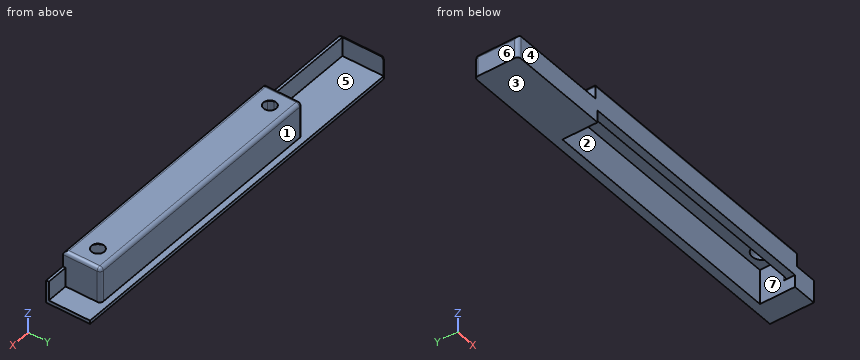
```python
from build123d import *

# Parameters (mm, degrees)
CROQUIS1_W                                   = 220
CROQUIS1_H                                   = 25
SALIENTE_EXTRUIR1_DEPTH                      = 2
SALIENTE_EXTRUIR2_DEPTH                      = 11
SALIENTE_EXTRUIR3_DEPTH                      = 7
CROQUIS5_W                                   = 150
CROQUIS5_H                                   = 20
SALIENTE_EXTRUIR4_DEPTH                      = 2
REDONDEO2_R                                  = 2
REDONDEO3_R                                  = 2
REDONDEO4_R                                  = 2
CROQUIS7_W                                   = 147
CROQUIS7_H                                   = 20
CORTAR_EXTRUIR1_DEPTH                        = 2
CROQUIS10_W                                  = 150
CROQUIS10_H                                  = 1.5
SALIENTE_EXTRUIR8_DEPTH                      = 15
CROQUIS11_R                                  = 2.25
CORTAR_EXTRUIR2_DEPTH                        = 15
REFRENTADO_PARA_TORNILLO_TAP_N_CON_C_2_COUNT = 2
REFRENTADO_PARA_TORNILLO_TAP_N_CON_C_2_PITCH = 128
REDONDEO5_R                                  = 2
CROQUIS14_W                                  = 147
CROQUIS14_H                                  = 3
SALIENTE_EXTRUIR9_DEPTH                      = 13
REDONDEO6_R                                  = 2


with BuildPart() as part:
    # Croquis1 → Saliente-Extruir1 (new body)
    with BuildSketch(Plane.XY):
        with Locations((-129.544939143, 51.184210526)):
            Rectangle(CROQUIS1_W, CROQUIS1_H)
    extrude(amount=SALIENTE_EXTRUIR1_DEPTH)

    # Croquis3 → Saliente-Extruir2 (add)
    with BuildSketch(Plane.XY.offset(2)):
        Polygon((-239.544939143, 63.684210526), (-239.544939143, 38.684210526), (-180.544939143, 38.684210526), (-180.544939143, 58.684210526), (-33.544939143, 58.684210526), (-33.544939143, 38.684210526), (-19.544939143, 38.684210526), (-19.544939143, 40.184210526), (-32.044939143, 40.184210526), (-32.044939143, 60.184210526), (-182.044939143, 60.184210526), (-182.044939143, 40.184210526), (-238.044939143, 40.184210526), (-238.044939143, 63.684210526), align=None)
    extrude(amount=SALIENTE_EXTRUIR2_DEPTH)

    # Croquis4 → Saliente-Extruir3 (add)
    with BuildSketch(Plane.XY.offset(13)):
        Polygon((-182.044939143, 40.184210526), (-180.544939143, 40.184210526), (-180.544939143, 40.470961068), (-180.544939143, 58.684210526), (-33.544939143, 58.684210526), (-33.544939143, 40.470961068), (-33.544939143, 40.184210526), (-32.044939143, 40.184210526), (-32.044939143, 40.470961068), (-32.044939143, 60.184210526), (-182.044939143, 60.184210526), align=None)
    extrude(amount=SALIENTE_EXTRUIR3_DEPTH)

    # Croquis5 → Saliente-Extruir4 (add)
    with BuildSketch(Plane.XY.offset(20)):
        with Locations((-107.044939143, 50.184210526)):
            Rectangle(CROQUIS5_W, CROQUIS5_H)
    extrude(amount=SALIENTE_EXTRUIR4_DEPTH)

    # Redondeo2
    redondeo2_edges = [part.edges().sort_by_distance(p)[0] for p in [
        (-239.544939143, 63.684210526, 6.5),
    ]]
    fillet(redondeo2_edges, radius=REDONDEO2_R)

    # Redondeo3
    # the kernel refuses this fillet: 2 mm, written as the material it takes off along each edge
    with BuildSketch(Plane(origin=(-239.544939143, 61.684210526, 13), x_dir=(1, 0, 0), z_dir=(0, -1, 0))) as redondeo3_piece_1:
        with BuildLine():
            CenterArc((REDONDEO3_R, -REDONDEO3_R), REDONDEO3_R, 90, 90)
            Line((0, -REDONDEO3_R), (0, 0))
            Line((0, 0), (REDONDEO3_R, 0))
        make_face()
    extrude(amount=28, mode=Mode.SUBTRACT)
    with BuildSketch(Plane(origin=(-237.544939143, 61.684210526, 13), x_dir=(0.7793111641702657, -0.6266371433290445, 0), z_dir=(-0.6266371433290445, -0.7793111641702657, 0))) as redondeo3_piece_2:
        with BuildLine():
            CenterArc((2 - REDONDEO3_R, -REDONDEO3_R), REDONDEO3_R, 0, 90)
            Line((2 - REDONDEO3_R, 0), (2, 0))
            Line((2, 0), (2, -REDONDEO3_R))
        make_face()
    revolve(axis=Axis((-237.544939143, 61.684210526, 13), (0, 0, 1)), revolution_arc=218.802450559, mode=Mode.SUBTRACT)

    # Redondeo4
    # the kernel refuses this fillet: 2 mm, written as the material it takes off along each edge
    with BuildSketch(Plane(origin=(-239.544939143, 38.684210526, -5), x_dir=(0, 1, 0), z_dir=(0, 0, 1))) as redondeo4_piece_1:
        with BuildLine():
            CenterArc((REDONDEO4_R, -REDONDEO4_R), REDONDEO4_R, 90, 90)
            Line((0, -REDONDEO4_R), (0, 0))
            Line((0, 0), (REDONDEO4_R, 0))
        make_face()
    extrude(amount=21, mode=Mode.SUBTRACT)

    # Croquis7 → Cortar-Extruir1 (cut)
    with BuildSketch(Plane.XY.offset(2)):
        with Locations((-107.044939143, 48.684210526)):
            Rectangle(CROQUIS7_W, CROQUIS7_H)
    extrude(amount=-CORTAR_EXTRUIR1_DEPTH, mode=Mode.SUBTRACT)

    # Croquis10 → Saliente-Extruir8 (add)
    with BuildSketch(Plane.XY.offset(22)):
        with Locations((-107.044939143, 39.434210526)):
            Rectangle(CROQUIS10_W, CROQUIS10_H)
    extrude(amount=-SALIENTE_EXTRUIR8_DEPTH)

    # Croquis11 → Cortar-Extruir2 (cut)
    with BuildSketch(Plane.XY.offset(22)):
        with Locations((-171.044939143, 50.184210526)):
            Circle(CROQUIS11_R)
        with Locations((-43.044939143, 50.184210526)):
            Circle(CROQUIS11_R)
    extrude(amount=-CORTAR_EXTRUIR2_DEPTH, mode=Mode.SUBTRACT)

    # Croquis12 → Refrentado para tornillo tapón con cabeza plana de clavija de M51 (revolve, cut)
    with BuildSketch(Plane(origin=(-171.044939143, 50.184210526, 20), x_dir=(0, 1, 0), z_dir=(1, 0, 0))):
        Polygon((0, 0), (0, 2), (2.9, 2), (2.9, 2.7), (5.6, 0), align=None)
    refrentado_para_tornillo_tap_n_con_cabez = revolve(axis=Axis((-171.044939143, 50.184210526, 13.65), (0, 0, 1)), mode=Mode.SUBTRACT)

    # Refrentado para tornillo tap_n con c 2: Refrentado para tornillo tapón con cabeza plana de clavija de M51 ×2
    with Locations(*[(i * REFRENTADO_PARA_TORNILLO_TAP_N_CON_C_2_PITCH, 0, 0) for i in range(1, REFRENTADO_PARA_TORNILLO_TAP_N_CON_C_2_COUNT)]):
        add(refrentado_para_tornillo_tap_n_con_cabez, mode=Mode.SUBTRACT)

    # Redondeo5
    redondeo5_edges = [part.edges().sort_by_distance(p)[0] for p in [
        (-107.044939143, 38.684210526, 22),
        (-32.044939143, 60.184210526, 12),
        (-182.044939143, 60.184210526, 12),
        (-182.044939143, 49.434210526, 22),
        (-32.044939143, 49.434210526, 22),
        (-107.044939143, 60.184210526, 22),
    ]]
    fillet(redondeo5_edges, radius=REDONDEO5_R)

    # Croquis14 → Saliente-Extruir9 (add)
    with BuildSketch(Plane(origin=(0, 0, 20), x_dir=(-1, 0, 0), z_dir=(0, 0, -1))):
        with Locations((107.044939143, 41.684210526)):
            Rectangle(CROQUIS14_W, CROQUIS14_H)
    extrude(amount=SALIENTE_EXTRUIR9_DEPTH)

    # Redondeo6
    redondeo6_edges = [part.edges().sort_by_distance(p)[0] for p in [
        (-180.544939143, 43.184210526, 13.5),
        (-107.044939143, 43.184210526, 20),
        (-33.544939143, 43.184210526, 13.5),
    ]]
    fillet(redondeo6_edges, radius=REDONDEO6_R)


solid = part.part
```
Geometry: final body of the model. Coordinates: model frame, mm. Face numbers are marked on the shaded views. A direction names the side the tool comes from. Round coordinates to 2 decimals unless told otherwise and drop trailing zeros. Loops run counter-clockwise (first coordinate to the right, second up) from the corner with the lowest first, then second, coordinate; pieces in that order, holes last. Notation, with made-up numbers: (-29, 55.5) -> (-15, 55.5) arc R16 cw to (-15, 86.5) -> close; hole circle Ø11 at (-8, -38.75). An arc over 180 degrees is marked (long way). Use one line per item in the form item = value.
Item 1: Cut plane C-C on z = 4.25. Output: boundary loops of the cut face in (x, y).
Evaluation:
outline = (-239.54, 40.68) arc R2 ccw to (-237.54, 38.68) -> (-180.54, 38.68) -> (-180.54, 58.68) -> (-33.54, 58.68) -> (-33.54, 38.68) -> (-19.54, 38.68) -> (-19.54, 40.18) -> (-32.04, 40.18) -> (-32.04, 58.18) arc R2 ccw to (-34.04, 60.18) -> (-180.04, 60.18) arc R2 ccw to (-182.04, 58.18) -> (-182.04, 40.18) -> (-238.04, 40.18) -> (-238.04, 63.62) arc R2 ccw to (-239.54, 61.68) -> close
Item 2: Cut plane A-A on z = 16. Output: boundary loops of the cut face in (x, y), then the cut area to 4 significant figures.
Evaluation:
outline = (-182.04, 38.68) -> (-32.04, 38.68) -> (-32.04, 58.18) arc R2 ccw to (-34.04, 60.18) -> (-180.04, 60.18) arc R2 ccw to (-182.04, 58.18) -> close; hole (-180.54, 45.18) arc R2 ccw to (-178.54, 43.18) -> (-35.54, 43.18) arc R2 ccw to (-33.54, 45.18) -> (-33.54, 58.68) -> (-180.54, 58.68) -> close
area = 946.5 mm2
Item 3: Cut plane B-B on x = -94.5. Output: boundary loops of the cut face in (y, z).
Evaluation:
outline = (38.68, 7) -> (43.18, 7) -> (43.18, 18) arc R2 cw to (45.18, 20) -> (58.68, 20) -> (58.68, 0) -> (63.68, 0) -> (63.68, 2) -> (60.18, 2) -> (60.18, 20) arc R2 ccw to (58.18, 22) -> (40.68, 22) arc R2 ccw to (38.68, 20) -> close
Item 4: Contact query for flat-ended pins moving along their axis: pin 1 Ø4 at (x, y) = (-115, 53) entering from -Z; pin 2 Ø3.5 at (x, z) = (-101.5, 10) entering from +Y; pin 3 Ø5.5 at (y, z) = (53, 8.5) entering from +X; pin 4 Ø8 at (x, y) = (-167.5, 50.5) entering from +Z. Output: stop coordinate, or through.
Evaluation:
pin_1 = 20
pin_2 = 60.18
pin_3 = -32.04
pin_4 = 22
Item 5: Material intervals for probe 1 along X at (y, z) = (57, 7.75); probe 2 along Y at (x, z) = (-88, 9.75); probe 3 along X at (y, z) = (57.25, 15), sorted ascending.
Evaluation:
probe_1 = -239.54 to -238.04, -182.04 to -180.54, -33.54 to -32.04
probe_2 = 38.68 to 43.18, 58.68 to 60.18
probe_3 = -182.04 to -180.54, -33.54 to -32.04
Item 6: Cut plane D-D on x = -187. Output: boundary loops of the cut face in (y, z).
Evaluation:
outline = (38.68, 0) -> (63.68, 0) -> (63.68, 2) -> (40.18, 2) -> (40.18, 13) -> (38.68, 13) -> close
Item 7: Access query for the marked faces 5, 6 and 7. Directions: +Z, -Z, +X, -X, +Y, -Y. A direction counts if a zero-diameter tool reaches every point of the face in a straight line with its end or side. Return the directions, or none.
Evaluation:
face_5 = +Z, +Y
face_6 = +Z, -Z, -X, +Y, -Y
face_7 = -Z
Item 8: Draft query along Y for the marked faces 1, 2, 3 and 4. Return one class per face: released by +Y, released by -Y, zero draft, split by the parting line, or undercut.
Evaluation:
face_1 = released by +Y
face_2 = undercut
face_3 = zero draft
face_4 = released by -Y
